Geometry check sheet. Reference: the model listing, model coordinates, mm. A direction names the side the tool comes from. Give positions to 0.01 mm unless a question says otherwise; leave off trailing zeros. Loops run counter-clockwise (first coordinate to the right, second up) from the corner with the lowest first, then second, coordinate; pieces in that order, holes last. Notation, with made-up numbers: (48, -39.75) -> (60, -39.75) arc R14 cw to (60, -12.75) -> close; hole circle Ø7 at (61, 45.5). An arc over 180 degrees is marked (long way). Answer as a JSON object with one key per item and string values.
from build123d import *

# Parameters (mm, degrees)
F0_W     = 50
F0_H     = 40
F1_DEPTH = 20
F2_SIZE  = 5
F4_DEPTH = 20
F6_DEPTH = 10


with BuildPart() as f1:
    # F0 (on Front) → F1 (new body)
    with BuildSketch(Plane.XZ):
        Rectangle(F0_W, F0_H)
    extrude(amount=F1_DEPTH)

    # F2
    f2_edges = [f1.edges().sort_by_distance(p)[0] for p in [
        (-25, -10, 20),
        (25, -10, 20),
        (-25, -10, -20),
        (25, -10, -20),
    ]]
    chamfer(f2_edges, length=F2_SIZE)

    # F3 (on face) → F4 (cut)
    with BuildSketch(Plane.XZ.offset(20)):
        with BuildLine():
            Line((-1, 7.3), (-4.8, 7.3))
            ThreePointArc((-4.8, 7.3), (-5.909619, 7.759619), (-5.45, 6.65))
            Line((-5.45, 6.65), (-5.45, -4.65))
            ThreePointArc((-5.45, -4.65), (-5.909619, -5.759619), (-4.8, -5.3))
            Line((-4.8, -5.3), (4.8, -5.3))
            ThreePointArc((4.8, -5.3), (5.909619, -5.759619), (5.45, -4.65))
            Line((5.45, -4.65), (5.45, 6.65))
            ThreePointArc((5.45, 6.65), (5.909619, 7.759619), (4.8, 7.3))
            Line((4.8, 7.3), (1, 7.3))
            Line((1, 7.3), (1, 9.3))
            ThreePointArc((1, 9.3), (0.707107, 10.007107), (0, 10.3))
            ThreePointArc((0, 10.3), (-0.707107, 10.007107), (-1, 9.3))
            Line((-1, 9.3), (-1, 7.3))
        make_face()
    extrude(amount=-F4_DEPTH, mode=Mode.SUBTRACT)

    # F5 (on face) → F6 (cut)
    with BuildSketch(Plane.XZ.offset(20)):
        with BuildLine():
            ThreePointArc((-6.3, -3.3), (-5.42132, -5.42132), (-3.3, -6.3))
            Line((-3.3, -6.3), (3.3, -6.3))
            ThreePointArc((3.3, -6.3), (5.42132, -5.42132), (6.3, -3.3))
            Line((6.3, -3.3), (6.3, 2.39))
            ThreePointArc((6.3, 2.39), (5.42132, 4.51132), (3.3, 5.39))
            Line((3.3, 5.39), (-3.3, 5.39))
            ThreePointArc((-3.3, 5.39), (-5.42132, 4.51132), (-6.3, 2.39))
            Line((-6.3, 2.39), (-6.3, -3.3))
        make_face()
    extrude(amount=-F6_DEPTH, mode=Mode.SUBTRACT)


solid = f1.part
1) Draft check along Z on faces 1 (the face through (23, -10, -17)), 2 (the face through (-6, -20, 5)), 3 (the face through (22, -10, 18)), 4 (the face through (6.3, -15, 0)). Enter one of: pulls with the +Z half, pulls with the -Z half, needs draft (parallel to the pull), parting line crosses it, or undercut.
Geometry check:
{"face 1": "pulls with the -Z half", "face 2": "needs draft", "face 3": "pulls with the +Z half", "face 4": "undercut"}
2) Material ranges on line 1 along X through (y, z) = (-15.5, -5.3); line 2 along Z through (x, y) = (4.5, -6.25); line 3 along X through (y, z) = (-13, -3), recorded low to high. Write a range as from..to.
Geometry check:
{"line 1": "x = -25..-6.1, 6.1..25", "line 2": "z = -20..-5.3, 7.3..20", "line 3": "x = -25..-6.3, 6.3..25"}
3) Tool access check on faces 5 (the face through (-1, -10, 8)), 6 (the face through (0, -10, 20)), 7 (the face through (-6.073, -15.07, 3.534)). Record the directions out of +Z, -Z, +X, -X, +Y, -Y that give a thin tool (end or side, any length) a straight path to the whole face; none if there is none.
Geometry check:
{"face 5": "+Y, -Y", "face 6": "+Z, +X, -X, +Y, -Y", "face 7": "-Y"}
4) Depth check by flat-ended pin: P1, Ø1.2, axis at x = 5.45, z = 7.3, coming from the -Y side. Enter the tip coordinate at first touch or a pass-through.
Geometry check:
{"P1": "passes through"}
5) Section check B-B on y = -3.5. Record the cut outline in (x, z), plus the area to 3 significant figures.
Geometry check:
{"outline": "(-25, -15) -> (-20, -20) -> (20, -20) -> (25, -15) -> (25, 15) -> (20, 20) -> (-20, 20) -> (-25, 15) -> close; hole (-5.45, -4.65) arc R0.65 ccw (long way) to (-4.8, -5.3) -> (4.8, -5.3) arc R0.65 ccw (long way) to (5.45, -4.65) -> (5.45, 6.65) arc R0.65 ccw (long way) to (4.8, 7.3) -> (1, 7.3) -> (1, 9.3) arc R1 ccw to (0, 10.3) arc R1 ccw to (-1, 9.3) -> (-1, 7.3) -> (-4.8, 7.3) arc R0.65 ccw (long way) to (-5.45, 6.65) -> close", "area": "1,800 mm2"}
